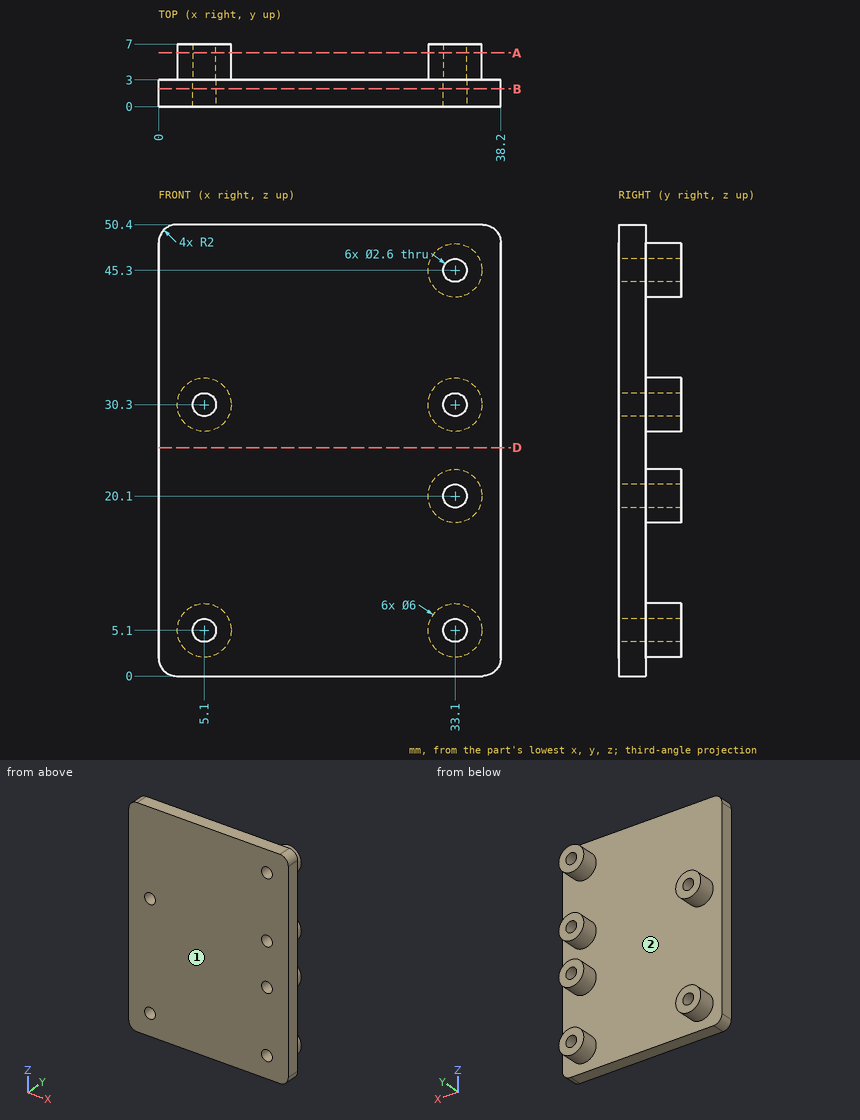
Input: dimensioned drawing with shaded views. Units: mm. Origin: part minimum x, y, z. Round coordinates to 2 decimals unless told otherwise and drop trailing zeros. Order: outer loops, then holes, each group sorted by start corner. A loop starts at its lowest first (then second) coordinate and runs counter-clockwise, first axis right, second up.
1. Pin query (flat end, axial travel): P1, Ø1.6, axis at x = 5.1, z = 30.3, coming from the +Y side; P2, Ø12, axis at x = 24.5, z = 25, coming from the +Y side. Return the tip coordinate at first contact, or that it passes through.
The answers:
P1: passes through
P2: stops at y = 3
2. Mould query, pull axis Z, two halves, no side actions, for the marked faces 1 and 2. Classes: released by +Z, released by -Z, zero draft, split by the parting line, or undercut.
The answers:
face 1: zero draft
face 2: undercut
3. Cut plane A-A, the plane y = 6. State how many separate pieces and enclosed holes the cut face has, then the cut area to 3 significant figures.
The answers:
separate pieces: 6
enclosed holes: 6
area: 138 mm2
4. Material intervals for line 1 (X direction, y = 4.5, z = 5.1); line 2 (Z direction, x = 5.1, y = 1.5); line 3 (Z direction, x = 33.1, y = 1.5), sorted ascending.
The answers:
line 1: x = 2.1 to 3.8, 6.4 to 8.1, 30.1 to 31.8, 34.4 to 36.1
line 2: z = 0 to 3.8, 6.4 to 29, 31.6 to 50.4
line 3: z = 0 to 3.8, 6.4 to 18.8, 21.4 to 29, 31.6 to 44, 46.6 to 50.4
5. Cut plane D-D, the plane z = 25.5. Output: boundary loops of the cut face in (x, y), then the cut area to 3 significant figures.
The answers:
outline: (0, 0) - (38.2, 0) - (38.2, 3) - (0, 3) - close
area: 115 mm2
6. Cut plane B-B, the plane y = 2. Output: boundary loops of the cut face in (x, z).
The answers:
outline: (0, 2) arc R2 ccw to (2, 0) - (36.2, 0) arc R2 ccw to (38.2, 2) - (38.2, 48.4) arc R2 ccw to (36.2, 50.4) - (2, 50.4) arc R2 ccw to (0, 48.4) - close; hole circle Ø2.6 at (5.1, 5.1); hole circle Ø2.6 at (5.1, 30.3); hole circle Ø2.6 at (33.1, 5.1); hole circle Ø2.6 at (33.1, 20.1); hole circle Ø2.6 at (33.1, 30.3); hole circle Ø2.6 at (33.1, 45.3)
